The model under review builds one solid part; all positions refer to its coordinate system, in mm. A direction names the side the tool comes from. Round coordinates to 2 decimals unless told otherwise and drop trailing zeros. Write each loop counter-clockwise with the first axis right and the second up, starting at its lowest first coordinate (ties: lowest second). Pieces come first, ordered by that corner, then holes. Notation, with made-up numbers: (-15, 74) -> (-8, 74) arc R11 ccw to (-8, 92) -> close; hole circle Ø3 at (88.5, 25). An arc over 180 degrees is marked (long way). Return JSON: item names as keys, results as strings. Group by question number.
1. Tool access review of faces 1 (the flat face through (3, 1, 2)), 2 (the cylindrical face through (6.686, 0.494, 0.323)): name each direction out of +Z, -Z, +X, -X, +Y, -Y from which nothing blocks a thin tool from reaching the whole face with its end or side.
2. Take a section at A-A, the plane x = 4.45. Write out the cut boundary in (y, z).
3. Take a section at C-C, the plane y = 1.85. Write out the cut boundary in (x, z).
4. Take a section at B-B, the plane z = 1.4. Write out the cut boundary in (x, y).
5. Take a section at D-D, the plane x = 6.25. Write out the cut boundary in (y, z), then the cut area to 3 significant figures.
6. For line 1 along X through (y, z) = (0.9, 1.1); line 2 along Y through (x, z) = (2.25, 1.45); line 3 along Y through (x, z) = (6, 0.35), list the stretches that pass through material, from the lowest coordinate up. Write a range as from..to.
7. Clearance check with a flat-ended pin moving along its axis: P1, Ø2, axis at x = 5.5, z = -1, coming from the -Y side. State where the tip first meets the part, or that it passes through.
from build123d import *

# Parameters (mm, degrees)
SKETCH1_W           = 5.7
SKETCH1_H           = 4
BOSS_EXTRUDE1_DEPTH = 2
SKETCH2_R           = 0.6
BOSS_EXTRUDE2_DEPTH = 2
SKETCH3_R           = 0.4
BOSS_EXTRUDE3_DEPTH = 0.6


# Read off the part's stored shape, not the designer's step: Dome1
with BuildPart() as part:
    # Sketch1 → Boss-Extrude1 (new body)
    with BuildSketch(Plane(origin=(0, 0, 0), x_dir=(1, 0, 0), z_dir=(0, 1, 0))):
        with Locations((2.85, 0)):
            Rectangle(SKETCH1_W, SKETCH1_H)
    extrude(amount=BOSS_EXTRUDE1_DEPTH)

    # Sketch2 → Boss-Extrude2 (add)
    with BuildSketch(Plane(origin=(5.7, 0, 0), x_dir=(0, 0, -1), z_dir=(1, 0, 0))):
        with Locations(Location((0, 1, 0), (0, 0, 180))):
            Circle(SKETCH2_R)
    extrude(amount=BOSS_EXTRUDE2_DEPTH)

    # Dome1 outline → Dome1 (revolve)
    with BuildSketch(Plane(origin=(0, 1, 0), x_dir=(0, 1, 0), z_dir=(0, 0, -1))):
        with BuildLine():
            add(Edge.make_bspline(
                [(0, 8.2), (0.6, 8.2), (0.6, 7.7)],
                knots=[4.71238898, 4.71238898, 4.71238898, 6.283185307, 6.283185307, 6.283185307], degree=2, weights=[1, 0.707106781, 1]))
            Line((0, 8.2), (0, 7.7))
            Line((0, 7.7), (0.6, 7.7))
        make_face()
    revolve(axis=Axis((0, 1, 0), (1, 0, 0)))

    # Sketch3 → Boss-Extrude3 (add)
    with BuildSketch(Plane(origin=(0, 0, 0), x_dir=(-1, 0, 0), z_dir=(0, -1, 0))):
        with Locations(Location((-4.45, 0, 0), (0, 0, 90))):
            Circle(SKETCH3_R)
        with Locations(Location((-1.45, 0, 0), (0, 0, 90))):
            Circle(SKETCH3_R)
    extrude(amount=BOSS_EXTRUDE3_DEPTH)


solid = part.part
Output:
{
 "1": {"face 1": "+Z, +X, -X, +Y, -Y", "face 2": "+X"},
 "2": {"outline": "(-0.6, -0.4) -> (0, -0.4) -> (0, -2) -> (2, -2) -> (2, 2) -> (0, 2) -> (0, 0.4) -> (-0.6, 0.4) -> close"},
 "3": {"outline": "(0, -2) -> (5.7, -2) -> (5.7, 2) -> (0, 2) -> close"},
 "4": {"outline": "(0, 0) -> (5.7, 0) -> (5.7, 2) -> (0, 2) -> close"},
 "5": {"outline": "circle Ø1.2 at (1, 0)", "area": "1.13 mm^2"},
 "6": {"line 1": "x = 0..5.7", "line 2": "y = 0..2", "line 3": "y = 0.51..1.49"},
 "7": {"P1": "stops at y = 0"}
}
